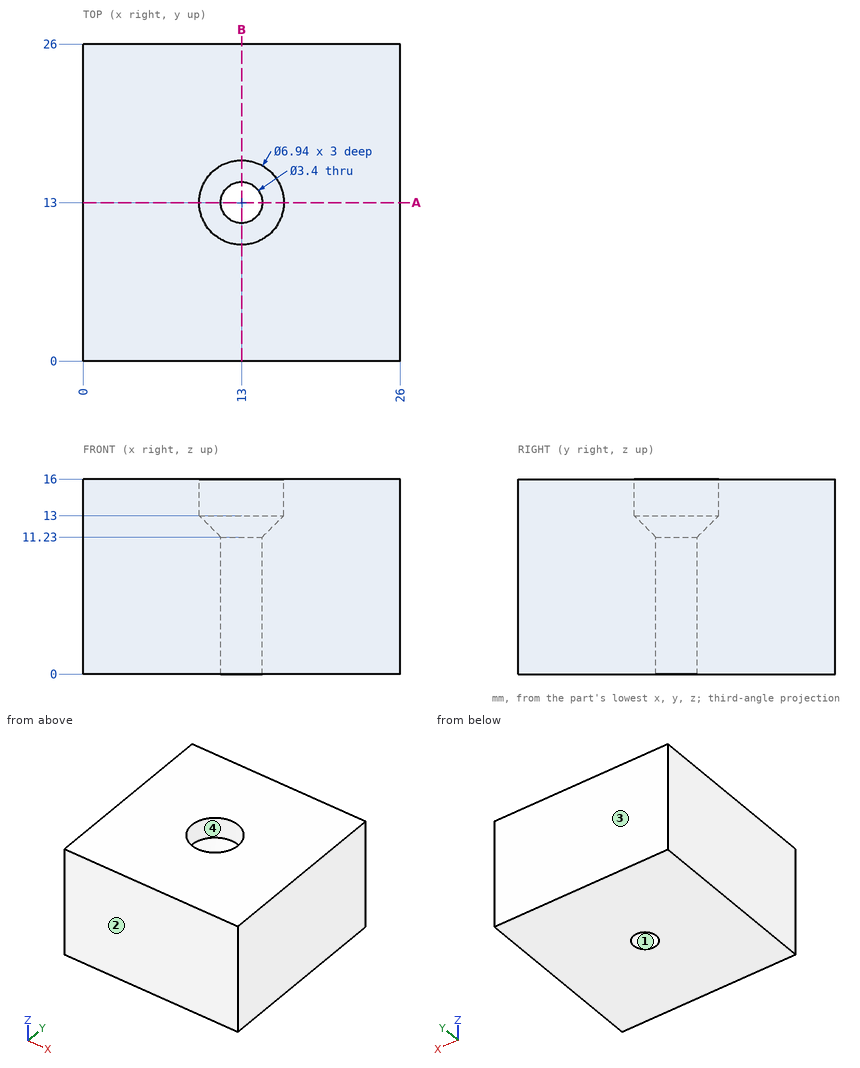
Study the drawing (mm; zero at the part's minimum x, y, z) and answer. Round coordinates to 2 decimals unless told otherwise and drop trailing zeros. Write each loop counter-clockwise with the first axis right and the second up, starting at its lowest first coordinate (ties: lowest second). Pieces come first, ordered by that corner, then holes. Notation, with made-up numbers: (38, -26) - (44, -26) arc R20 cw to (44, 4) - close; hole circle Ø5 at (48.5, -3). An arc over 180 degrees is marked (long way). Use CSV: the item, a comma, the result in double quotes.
Q1. Determine the mould class of the marked faces 1, 2, 3 and 4 for opening direction Y: +Y half, -Y half, draft (parallel to the pull), parting line (faces both ways), or undercut.
Values:
face 1,"undercut"
face 2,"-Y half"
face 3,"+Y half"
face 4,"undercut"
Q2. Straight lines are drawn through the part: line 1 along X through (y, z) = (13, 14.9); line 2 along X through (y, z) = (13, 5.5). For each, find the intervals that lie inside material, in ascending order.
Values:
line 1,"x = 0 to 9.53, 16.47 to 26"
line 2,"x = 0 to 11.3, 14.7 to 26"
Q3. Find section A-A, the plane y = 13. Write down the section's boundary in (x, z), then the cut area to 3 significant figures.
Values:
outline,"(0, 0) - (11.3, 0) - (11.3, 11.23) - (9.53, 13) - (9.53, 16) - (0, 16) - close; (14.7, 0) - (26, 0) - (26, 16) - (16.47, 16) - (16.47, 13) - (14.7, 11.23) - close"
area,"348 mm²"
Q4. Each of these flat-tipped pins is pushed along its axis until it touches: pin 1 Ø5 at (x, z) = (3, 8) entering from -Y; pin 2 Ø6 at (x, y) = (13, 13) entering from +Z. Where does it stop, or does it pass through?
Values:
pin 1,"stops at y = 0"
pin 2,"stops at z = 12.53"
